```python
from build123d import *

# Parameters (mm, degrees)
F0_R     = 7.6
F1_DEPTH = 1.6
F2_R     = 2.85
F3_DEPTH = 3
F4_R     = 1.5
F5_DEPTH = 25
F6_SIZE  = 0.5


with BuildPart() as f1:
    # F0 (on Top) → F1 (new body)
    with BuildSketch(Plane.XY):
        Circle(F0_R)
    extrude(amount=F1_DEPTH)

    # F2 (on face) → F3 (join)
    with BuildSketch(Plane.XY.offset(1.6)):
        Circle(F2_R)
    extrude(amount=F3_DEPTH)

    # F4 (on face) → F5 (cut)
    with BuildSketch(Plane.XY.offset(4.6)):
        Circle(F4_R)
    extrude(amount=-F5_DEPTH, mode=Mode.SUBTRACT)

    # F6
    f6_edges = [f1.edges().sort_by_distance(p)[0] for p in [
        (-1.5, 0, 0),
    ]]
    chamfer(f6_edges, length=F6_SIZE)


solid = f1.part
```
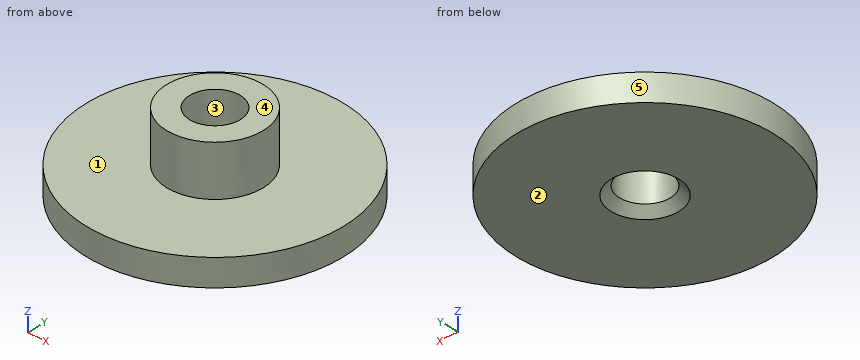
Work out the finished part from the listing and answer in its coordinate system (mm). Face numbers are marked on the shaded views. A direction names the side the tool comes from. Coordinates: 2 decimals unless noted, no trailing zeros. Order: outer loops, then holes, each group sorted by start corner. A loop starts at its lowest first (then second) coordinate and runs counter-clockwise, first axis right, second up. Notation, with made-up numbers: M 23.5,-35 L 47.5,-35 A9 cw 47.5,-31 Z; hole C -1,46 d9. An arc over 180 degrees is marked long. Use CSV: the item, a comma, the result in double quotes.
1) For the marked faces 1 and 2, determine the directions among +Z, -Z, +X, -X, +Y, -Y from which every point of the face is accessible in a straight line to the end or side of a thin tool.
Worked out:
face 1,"+Z"
face 2,"-Z, +X, -X, +Y, -Y"
2) Section D-D on x = -2.5 is taken. Write down the section's boundary in (y, z).
Worked out:
outline,"M -7.18,0 L 7.18,0 L 7.18,1.6 L 1.37,1.6 L 1.37,4.6 L -1.37,4.6 L -1.37,1.6 L -7.18,1.6 Z"
3) Section A-A on x = 0 is taken. Write down the section's boundary in (y, z).
Worked out:
outline,"M -7.6,0 L -2,0 L -1.5,0.5 L -1.5,4.6 L -2.85,4.6 L -2.85,1.6 L -7.6,1.6 Z; M 1.5,0.5 L 2,0 L 7.6,0 L 7.6,1.6 L 2.85,1.6 L 2.85,4.6 L 1.5,4.6 Z"
4) Flat-ended cylindrical pins translate along their axes: pin 1 Ø1.5 at (x, z) = (-1, 2.5) entering from +Y; pin 2 Ø2.5 at (x, y) = (0, 0) entering from -Z. Find the tip coordinate at first contact, or state that the pin passes through.
Worked out:
pin 1,"stops at y = 2.84"
pin 2,"passes through"
5) Consider line 1 (Y direction, x = 0, z = 2.85); line 2 (Y direction, x = 1.25, z = 0.4); line 3 (Z direction, x = 3.25, y = 2.25). Determine where each line is inside the solid, lowest interval first. Write a range as [from, to].
Worked out:
line 1,"y = [-2.85, -1.5], [1.5, 2.85]"
line 2,"y = [-7.5, -1], [1, 7.5]"
line 3,"z = [0, 1.6]"
6) Section C-C on z = 0.9 is taken. Write down the section's boundary in (x, y), plus the area to 3 significant figures.
Worked out:
outline,"C 0,0 d15.2; hole C 0,0 d3"
area,"174 mm^2"
7) Determine the mould class of the marked faces 3, 4 and 5 for opening direction Y: released by +Y, released by -Y, zero draft, split by the parting line, or undercut.
Worked out:
face 3,"undercut"
face 4,"zero draft"
face 5,"split by the parting line"
